The model under review builds one solid part; all positions refer to its coordinate system, in mm. Face numbers are marked on the shaded views. A direction names the side the tool comes from. Coordinates: 2 decimals unless noted, no trailing zeros. Loops run counter-clockwise (first coordinate to the right, second up) from the corner with the lowest first, then second, coordinate; pieces in that order, holes last. Notation, with made-up numbers: M -13,3 L 20,3 A16 ccw 20,34 Z; hole C 29.5,4 d2. An arc over 180 degrees is marked long. Use CSV: the item, a comma, the result in double quotes. Start each with the question number.
1. Add section B-B, the plane y = -8. Write out the cut boundary in (x, z).
2. Add section C-C, the plane z = 6. Write out the cut boundary in (x, y), then the cut area to 3 significant figures.
3. Draft analysis for pull direction Y (two halves, no side actions). For the marked faces 1, 2 and 3, state which applies: +Y half, -Y half, draft (parallel to the pull), parting line (faces both ways), or undercut.
4. Clearance check with flat-ended pins moving along their axes: P1, Ø12, axis at x = 161, y = -7.5, coming from the +Z side; P2, Ø5, axis at y = -7.5, z = 3, coming from the -X side. State where each tip first meets the part, or that it passes through.
5. Add section A-A, the plane x = 154. Write out the cut boundary in (y, z), then the cut area to 3 significant figures.
6. Add section D-D, the plane y = -3.5. Write out the cut boundary in (x, z).
7. For L1, parallel to Y at x = 194.5, z = 3; L2, parallel to Y at x = 172, z = 10.5; L3, parallel to X at y = -3.5, z = 9, list the stretches that pass through material, from the lowest coordinate up.
8. Tool access review of the marked faces 4 and 5: name each direction out of +Z, -Z, +X, -X, +Y, -Y from which nothing blocks a thin tool from reaching the whole face with its end or side.
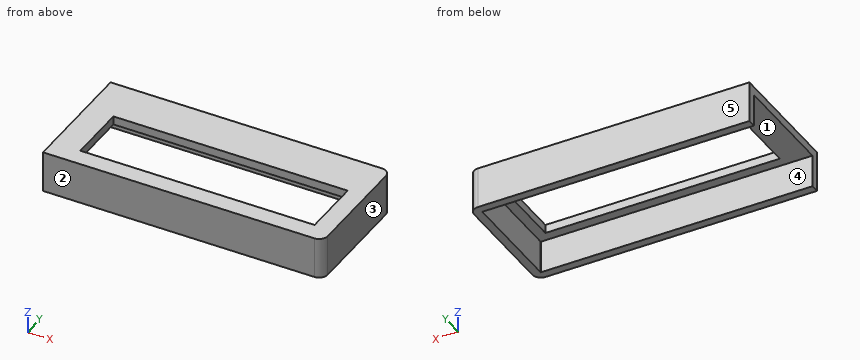
from build123d import *

# Parameters (mm, degrees)
PAD038_DEPTH    = 9.55
THICKNESS004_T  = -2.4
SKETCH044_W     = 30.9
SKETCH044_H     = 9.55
POCKET008_DEPTH = 2.4
SKETCH040_W     = 68.5
SKETCH040_H     = 17.5
PAD036_DEPTH    = 2.5


with BuildPart() as body012:
    # Sketch043 → Pad038 (new body)
    with BuildSketch(Plane.XY):
        with BuildLine():
            Line((126.75, 6.7), (126.75, -29))
            Line((126.75, -29), (206.1, -29))
            ThreePointArc((206.1, -29), (207.867767, -28.267767), (208.6, -26.5))
            Line((208.6, -26.5), (208.6, 4.2))
            ThreePointArc((208.6, 4.2), (207.867767, 5.967767), (206.1, 6.7))
            Line((206.1, 6.7), (126.75, 6.7))
        make_face()
    extrude(amount=-PAD038_DEPTH)

    # Thickness004
    thickness004_openings = [body012.faces().sort_by_distance(p)[0] for p in [
        (167.637908, -11.15, -9.55),
        (167.637908, -11.15, 0),
    ]]
    offset(amount=THICKNESS004_T, openings=thickness004_openings, kind=Kind.INTERSECTION)

    # Sketch044 (on Face8 of Thickness004) → Pocket008 (cut)
    with BuildSketch(Plane.YZ.offset(129.15)):
        with Locations((-11.15, -4.775)):
            Rectangle(SKETCH044_W, SKETCH044_H)
    extrude(amount=-POCKET008_DEPTH, mode=Mode.SUBTRACT)


with BuildPart() as body012_1:
    # Body012 placement: moved
    add(body012.part.moved(Location((0, 0, 10))))


with BuildPart() as tail_cover:
    # Sketch040 → Pad036 (new body)
    with BuildSketch(Plane.XY):
        with BuildLine():
            Line((126.75, 6.7), (126.75, -29))
            Line((126.75, -29), (206.1, -29))
            ThreePointArc((206.1, -29), (207.867767, -28.267767), (208.6, -26.5))
            Line((208.6, -26.5), (208.6, 4.2))
            ThreePointArc((208.6, 4.2), (207.867767, 5.967767), (206.1, 6.7))
            Line((206.1, 6.7), (126.75, 6.7))
        make_face()
        with Locations((169, -15)):
            Rectangle(SKETCH040_W, SKETCH040_H, mode=Mode.SUBTRACT)
    extrude(amount=PAD036_DEPTH)


with BuildPart() as tail_cover_1:
    # Body010 placement: moved
    add(tail_cover.part.moved(Location((0, 0, 10))))

    # Fusion: union Body012
    add(body012_1.part)


with BuildPart() as tail_cover_2:
    # Fusion placement: moved
    add(tail_cover_1.part.moved(Location((0, 0, -0.45))))


solid = tail_cover_2.part
Computed:
1,outline,"M 126.75,9.55 L 134.75,9.55 L 134.75,12.05 L 126.75,12.05 Z; M 203.25,9.55 L 206.2,9.55 L 206.2,0 L 208.6,0 L 208.6,12.05 L 203.25,12.05 Z"
2,outline,"M 126.75,-29 L 206.1,-29 A2.5 ccw 208.6,-26.5 L 208.6,4.2 A2.5 ccw 206.1,6.7 L 126.75,6.7 L 126.75,4.3 L 206.1,4.3 A0.1 cw 206.2,4.2 L 206.2,-26.5 A0.1 cw 206.1,-26.6 L 126.75,-26.6 Z"
2,area,"464 mm^2"
3,face 1,"undercut"
3,face 2,"-Y half"
3,face 3,"draft"
4,P1,"stops at z = 12.05"
4,P2,"stops at x = 206.2"
5,outline,"M -29,0 L -26.6,0 L -26.6,9.55 L -23.75,9.55 L -23.75,12.05 L -29,12.05 Z; M -6.25,9.55 L 4.3,9.55 L 4.3,0 L 6.7,0 L 6.7,12.05 L -6.25,12.05 Z"
5,area,"91.3 mm^2"
6,outline,"M 126.75,9.55 L 206.2,9.55 L 206.2,0 L 208.6,0 L 208.6,12.05 L 126.75,12.05 Z"
7,L1,"y = -29 to -26.6, 4.3 to 6.7"
7,L2,"y = -29 to -23.75, -6.25 to 6.7"
7,L3,"x = 206.2 to 208.6"
8,face 4,"-Z, -X"
8,face 5,"+Z, -Z, +X, -X, +Y"
